```python
from build123d import *

# Parameters (mm, degrees)
SKETCH1_R           = 1.7272
BOSS_EXTRUDE1_DEPTH = 5.9055
SKETCH6_R           = 5.1816
CUT_EXTRUDE4_DEPTH  = 22.094195358


with BuildPart() as part:
    # Sketch1 → Boss-Extrude1 (new body)
    with BuildSketch(Plane(origin=(0, 0, 0), x_dir=(1, 0, 0), z_dir=(0, 1, 0))):
        with BuildLine():
            Line((-15.0296372, 2.004639139), (-9.6266, 8.283632805))
            ThreePointArc((-9.6266, 8.283632805), (0, 12.7), (9.6266, 8.283632805))
            Line((9.6266, 8.283632805), (15.0296372, 2.004639139))
            ThreePointArc((15.0296372, 2.004639139), (15.7734, 0), (15.0296372, -2.004639139))
            Line((15.0296372, -2.004639139), (9.6266, -8.283632805))
            ThreePointArc((9.6266, -8.283632805), (0, -12.7), (-9.6266, -8.283632805))
            Line((-9.6266, -8.283632805), (-15.0296372, -2.004639139))
            ThreePointArc((-15.0296372, -2.004639139), (-15.7734, 0), (-15.0296372, 2.004639139))
        make_face()
        with Locations(Location((-12.7, 0, 0), (0, 0, 270))):
            Circle(SKETCH1_R, mode=Mode.SUBTRACT)
        with Locations(Location((12.7, 0, 0), (0, 0, 270))):
            Circle(SKETCH1_R, mode=Mode.SUBTRACT)
    extrude(amount=BOSS_EXTRUDE1_DEPTH)

    # Sketch6 → Cut-Extrude4 (cut, through all)
    with BuildSketch(Plane(origin=(0, 5.9055, 0), x_dir=(1, 0, 0), z_dir=(0, 1, 0))):
        with Locations(Location((0, 0, 0), (0, 0, 270))):
            Circle(SKETCH6_R)
    extrude(amount=-CUT_EXTRUDE4_DEPTH, mode=Mode.SUBTRACT)


solid = part.part
```
Verification items for the finished model (mm, model axes). Round coordinates to 2 decimals unless told otherwise and drop trailing zeros. Order: outer loops, then holes, each group sorted by start corner. A loop starts at its lowest first (then second) coordinate and runs counter-clockwise, first axis right, second up.
1) Cross-section at D-D, the plane x = -12.7. Record the cut outline in (y, z), plus the area to 3 significant figures.
Geometry says:
outline: (0, -4.71) - (5.91, -4.71) - (5.91, -1.73) - (0, -1.73) - close; (0, 1.73) - (5.91, 1.73) - (5.91, 4.71) - (0, 4.71) - close
area: 35.3 mm2
2) Material ranges on line 1 (X direction, y = 5.4, z = 0.5); line 2 (Z direction, x = -12.5, y = 2.4); line 3 (X direction, y = 3.6, z = -1), recorded low to high.
Geometry says:
line 1: x = -15.73 to -14.35, -11.05 to -5.16, 5.16 to 11.05, 14.35 to 15.73
line 2: z = -4.94 to -1.72, 1.72 to 4.94
line 3: x = -15.61 to -14.11, -11.29 to -5.08, 5.08 to 11.29, 14.11 to 15.61
3) Cross-section at B-B, the plane x = 0. Record the cut outline in (y, z).
Geometry says:
outline: (0, -12.7) - (5.91, -12.7) - (5.91, -5.18) - (0, -5.18) - close; (0, 5.18) - (5.91, 5.18) - (5.91, 12.7) - (0, 12.7) - close
4) Cross-section at A-A, the plane z = 0. Record the cut outline in (x, y), plus the area to 3 significant figures.
Geometry says:
outline: (-15.77, 0) - (-14.43, 0) - (-14.43, 5.91) - (-15.77, 5.91) - close; (-10.97, 0) - (-5.18, 0) - (-5.18, 5.91) - (-10.97, 5.91) - close; (5.18, 0) - (10.97, 0) - (10.97, 5.91) - (5.18, 5.91) - close; (14.43, 0) - (15.77, 0) - (15.77, 5.91) - (14.43, 5.91) - close
area: 84.3 mm2
5) Depth check by flat-ended pin: pin 1 (5.5 mm diameter, centred on x = -12.7, z = 0, fed in from -Y); pin 2 (3 mm diameter, centred on y = 5, z = 10, fed in from +X); pin 3 (1 mm diameter, centred on y = 2, z = -8, fed in from -X). Enter the tip coordinate at first touch or a pass-through.
Geometry says:
pin 1: stops at y = 0
pin 2: stops at x = 9.44
pin 3: stops at x = -10.3
6) Cross-section at C-C, the plane y = 1.15. Record the cut outline in (x, z).
Geometry says:
outline: (-15.03, -2) - (-9.63, -8.28) arc R12.7 ccw to (9.63, -8.28) - (15.03, -2) arc R3.07 ccw to (15.03, 2) - (9.63, 8.28) arc R12.7 ccw to (-9.63, 8.28) - (-15.03, 2) arc R3.07 ccw to start; hole circle Ø3.45 at (-12.7, 0); hole circle Ø10.36 at (0, 0); hole circle Ø3.45 at (12.7, 0)
